Autodesk Inventor part; units mm, degrees
ref_plane "YZ Plane" through (0, 0, 0) normal (1, 0, 0) x (0, 1, 0)
ref_plane "XZ Plane" through (0, 0, 0) normal (0, 1, 0) x (-1, 0, 0)
ref_plane "XY Plane" through (0, 0, 0) normal (0, 0, 1) x (1, 0, 0)
sketch "Sketch1" plane through (0, 0, 0) normal (0, 0, 1) x (1, 0, 0)
  line L0 (-6.5, -16) -> (6.5, -16)
  line L1 (6.5, -16) -> (6.5, 16)
  line L2 (6.5, 16) -> (-6.5, 16)
  line L3 (-6.5, 16) -> (-6.5, -16)
  line L4 (-6.5, -16) -> (6.5, 16) construction
  line L5 (6.5, -16) -> (-6.5, 16) construction
  line L6 (0, 0) -> (0, 12.5) construction
  line L7 (0, 0) -> (0, -12.5) construction
  circle A0 centre (0, 12.5) radius 1.65
  circle A1 centre (0, -12.5) radius 1.65
  dimension "d0" = 13
  dimension "d1" = 32
  dimension "d8" = 3.3
  dimension "d9" = 25
extrude "Extrusion1" add sketch "Sketch1" along normal blind 1.5
fillet "Fillet1" radius 2 4 edges at (6.5, 16, 0.75) (-6.5, 16, 0.75) (-6.5, -16, 0.75) (6.5, -16, 0.75)
sketch "Sketch2" plane through (0, 0, 1.5) normal (0, 0, 1) x (1, 0, 0)
  line L0 (6.5, -14) -> (6.5, 14)
  line L1 (6.5, -9) -> (9.5, -9)
  line L2 (9.5, -9) -> (9.5, -14)
  line L3 (9.5, -14) -> (6.5, -14) construction
  line L4 (9.5, -14) -> (13.5, -14)
  line L5 (13.5, -14) -> (13.5, -7)
  line L6 (13.5, -7) -> (6.5, 5.1244)
  line L7 (0, 0) -> (0, -8.4482) construction
  line L8 (6.5, 5.1244) -> (6.5, -9)
  line L9 (-6.5, -9) -> (-9.5, -9)
  line L10 (-9.5, -9) -> (-9.5, -14)
  line L11 (-9.5, -14) -> (-6.5, -14) construction
  line L12 (-9.5, -14) -> (-13.5, -14)
  line L13 (-13.5, -14) -> (-13.5, -7)
  line L14 (-13.5, -7) -> (-6.5, 5.1244)
  line L15 (-6.5, 5.1244) -> (-6.5, -9)
  dimension "d10" = 3
  dimension "d11" = 5
  dimension "d12" = 4
  dimension "d13" = 2
  dimension "d14" = 30
extrude "Extrusion2" add sketch "Sketch2" against normal blind 1.5
properties part number "PusherConstraint"
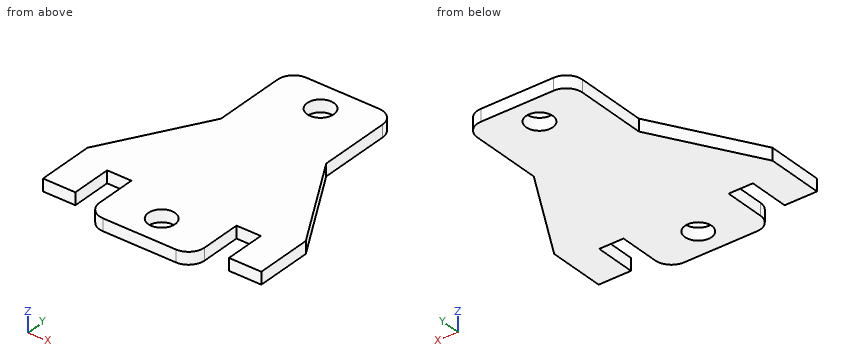
Model file for the job. Use its own axes, mm. Coordinates: 2 decimals unless noted, no trailing zeros. Order: outer loops, then holes, each group sorted by start corner. A loop starts at its lowest first (then second) coordinate and runs counter-clockwise, first axis right, second up. Notation, with made-up numbers: (5.5, 4) -> (11.5, 4) arc R23 cw to (11.5, 29) -> close; hole circle Ø4 at (83, 22.5). An arc over 180 degrees is marked (long way). Return JSON: item names as keys, results as strings.
Item 1: Slice it at D-D (z = 0.4). Write the cut outline in (x, y), then the cut area to 3 significant figures.
Model answer:
{"outline": "(-13.5, -14) -> (-9.5, -14) -> (-9.5, -9) -> (-6.5, -9) -> (-6.5, -14) arc R2 ccw to (-4.5, -16) -> (4.5, -16) arc R2 ccw to (6.5, -14) -> (6.5, -9) -> (9.5, -9) -> (9.5, -14) -> (13.5, -14) -> (13.5, -7) -> (6.5, 5.12) -> (6.5, 14) arc R2 ccw to (4.5, 16) -> (-4.5, 16) arc R2 ccw to (-6.5, 14) -> (-6.5, 5.12) -> (-13.5, -7) -> close; hole circle Ø3.3 at (0, -12.5); hole circle Ø3.3 at (0, 12.5)", "area": "548 mm²"}
Item 2: Pin check, flat tips, straight feed: P1, Ø5.5, axis at x = 0, y = 12.5, coming from the +Z side; P2, Ø0.8, axis at x = -7.5, z = 0.5, coming from the -Y side. Stop position of each tip, or through.
Model answer:
{"P1": "stops at z = 1.5", "P2": "stops at y = -9"}
Item 3: Slice it at B-B (x = 0). Write the cut outline in (y, z), then the cut area to 3 significant figures.
Model answer:
{"outline": "(-16, 0) -> (-14.15, 0) -> (-14.15, 1.5) -> (-16, 1.5) -> close; (-10.85, 0) -> (10.85, 0) -> (10.85, 1.5) -> (-10.85, 1.5) -> close; (14.15, 0) -> (16, 0) -> (16, 1.5) -> (14.15, 1.5) -> close", "area": "38.1 mm²"}
Item 4: Wall check: line 1 along Y through (x, z) = (0, 0.45); line 2 along X through (y, z) = (6, 0.3); line 3 along X through (y, z) = (2.5, 0.6). Give the ranges that are in metal, low to high. Write a range as from..to.
Model answer:
{"line 1": "y = -16..-14.15, -10.85..10.85, 14.15..16", "line 2": "x = -6.5..6.5", "line 3": "x = -8.02..8.02"}
Item 5: Slice it at C-C (y = 12.5). Write the cut outline in (x, z), then the cut area to 4 significant figures.
Model answer:
{"outline": "(-6.5, 0) -> (-1.65, 0) -> (-1.65, 1.5) -> (-6.5, 1.5) -> close; (1.65, 0) -> (6.5, 0) -> (6.5, 1.5) -> (1.65, 1.5) -> close", "area": "14.55 mm²"}
Item 6: Slice it at A-A (y = -12.5). Write the cut outline in (x, z).
Model answer:
{"outline": "(-13.5, 0) -> (-9.5, 0) -> (-9.5, 1.5) -> (-13.5, 1.5) -> close; (-6.5, 0) -> (-1.65, 0) -> (-1.65, 1.5) -> (-6.5, 1.5) -> close; (1.65, 0) -> (6.5, 0) -> (6.5, 1.5) -> (1.65, 1.5) -> close; (9.5, 0) -> (13.5, 0) -> (13.5, 1.5) -> (9.5, 1.5) -> close"}
